For this review, take the finished solid that the model builds, in its own axes (mm). Face numbers are marked on the shaded views. Coordinates: 2 decimals unless noted, no trailing zeros. Loops run counter-clockwise (first coordinate to the right, second up) from the corner with the lowest first, then second, coordinate; pieces in that order, holes last. Notation, with made-up numbers: (56.25, 41.25) - (111.25, 41.25) arc R20 cw to (111.25, 78.25) - close; hole circle Ø5 at (-11, 27.5). An arc over 180 degrees is marked (long way). One line per item, written item: value. Start each with the question number.
1. The part is to be moulded in two halves that separate along Y. For the marked faces 1, 2 and 3, say which applies: released by +Y, released by -Y, zero draft, split by the parting line, or undercut.
2. To check wall thickness, follow line 1 (Y direction, x = 0, z = 1.75); line 2 (X direction, y = -1, z = 2.85); line 3 (X direction, y = 1.25, z = 1.1). State the ranges of each line that lie inside material, in increasing order. Write a range as from..to.
3. Take a section at C-C, the plane z = 1.5. State the section outline as (x, y) points, and give its area (3 significant figures).
4. Take a section at A-A, the plane x = 0. State the section outline as (y, z) points, and give its area (3 significant figures).
5. Insertion check: pin 1 (4 mm diameter, centred on x = 3.5, y = 2, fed in from +Z); pin 2 (1.5 mm diameter, centred on x = 3.5, z = 2.5, fed in from -Y). Each pin has a flat end and moves straight along its axis. Give the tip position at first contact, or say it passes through.
6. Take a section at B-B, the plane y = 1.5. State the section outline as (x, z) points, and give its area (3 significant figures).
7. Take a section at D-D, the plane x = -3.25. State the section outline as (y, z) points.
```python
from build123d import *

# Parameters (mm, degrees)
F0_R     = 2.0447
F1_DEPTH = 3.048
F2_SIZE  = 0.381


with BuildPart() as f1:
    # F0 (on Top) → F1 (new body)
    with BuildSketch(Plane.XY):
        Polygon((-2.456337, -4.2545), (2.456337, -4.2545), (4.912673, 0), (2.456337, 4.2545), (-2.456337, 4.2545), (-4.912673, 0), align=None)
        Circle(F0_R, mode=Mode.SUBTRACT)
    extrude(amount=F1_DEPTH)

    # F2
    f2_edges = [f1.edges().sort_by_distance(p)[0] for p in [
        (3.684505, -2.12725, 3.048),
        (0, -4.2545, 3.048),
        (-3.684505, -2.12725, 3.048),
        (-3.684505, 2.12725, 3.048),
        (0, 4.2545, 3.048),
        (3.684505, 2.12725, 3.048),
        (0, -4.2545, 0),
        (-3.684505, -2.12725, 0),
        (3.684505, -2.12725, 0),
        (3.684505, 2.12725, 0),
        (0, 4.2545, 0),
        (-3.684505, 2.12725, 0),
    ]]
    chamfer(f2_edges, length=F2_SIZE)


solid = f1.part
```
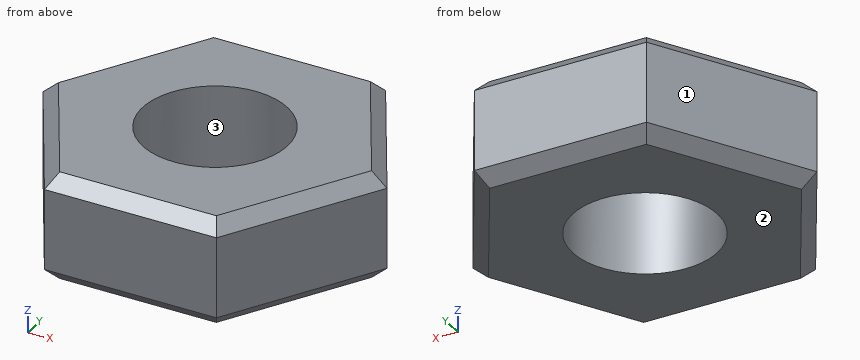
Solutions:
1. face 1: released by +Y
1. face 2: zero draft
1. face 3: undercut
2. line 1: -4.25..-2.04, 2.04..4.25
2. line 2: -4.12..-1.78, 1.78..4.12
2. line 3: -4.19..-1.62, 1.62..4.19
3. outline: (-4.91, 0) - (-2.46, -4.25) - (2.46, -4.25) - (4.91, 0) - (2.46, 4.25) - (-2.46, 4.25) - close; hole circle Ø4.09 at (0, 0)
3. area: 49.6 mm2
4. outline: (-4.25, 0.38) - (-3.87, 0) - (-2.04, 0) - (-2.04, 3.05) - (-3.87, 3.05) - (-4.25, 2.67) - close; (2.04, 0) - (3.87, 0) - (4.25, 0.38) - (4.25, 2.67) - (3.87, 3.05) - (2.04, 3.05) - close
4. area: 13.2 mm2
5. pin 1: z = 3.05
5. pin 2: y = -3.75
6. outline: (-4.05, 0.38) - (-3.61, 0) - (-1.39, 0) - (-1.39, 3.05) - (-3.61, 3.05) - (-4.05, 2.67) - close; (1.39, 0) - (3.61, 0) - (4.05, 0.38) - (4.05, 2.67) - (3.61, 3.05) - (1.39, 3.05) - close
6. area: 15.9 mm2
7. outline: (-2.88, 0.38) - (-2.12, 0) - (2.12, 0) - (2.88, 0.38) - (2.88, 2.67) - (2.12, 3.05) - (-2.12, 3.05) - (-2.88, 2.67) - close
